Build history of the part. All positions in model axes, mm. Face numbers are marked on the shaded views. A direction names the side the tool comes from. Give positions to 0.01 mm unless a question says otherwise; leave off trailing zeros. Write each loop counter-clockwise with the first axis right and the second up, starting at its lowest first coordinate (ties: lowest second). Pieces come first, ordered by that corner, then holes. Notation, with made-up numbers: M 62.25,-28.5 L 69.25,-28.5 A26 cw 69.25,8.5 Z; hole C -11.75,19 d8. An arc over 180 degrees is marked long. Return JSON: item names as keys, results as strings. Group by question number.
Q1. Band-saw the part on A-A, the plane y = -16.75. Give the cut face in (x, z) (3 decimals), then the cut area to 3 significant figures.
Q2. Band-saw the part on C-C, the plane y = -7.62. Give the cut face in (x, z) (3 decimals), then the cut area to 3 significant figures.
Q3. Band-saw the part on B-B, the plane z = -3.5. Give the cut face in (x, y) (3 decimals).
Q4. Tool access for the marked faces 5 and 6: list every direction of +Z, -Z, +X, -X, +Y, -Y with a clear straight run to the whole face (end or side of a thin tool).
Q5. Band-saw the part on D-D, the plane x = 6. Give the cut face in (y, z).
Q6. Flat gauge pins, fed straight in: pin 1 Ø1.6 at (x, y) = (62, -12.5) entering from -Z; pin 2 Ø1 at (y, z) = (-15, -25.5) entering from -X; pin 3 Ø3 at (y, z) = (-6.5, -34.5) entering from +X (3 decimals). Where does each tip first touch, or does it go through?
Q7. Wall check: probe 1 along X at (y, z) = (-7.62, -9.75); probe 2 along X at (y, z) = (-6.25, -18); probe 3 along Z at (x, y) = (41.5, -1.5). Give the ranges that are in metal, low to high.
Q8. Pull direction Y, two halves, no side cores. Call the marked faces 1, 2, 3 and 4: +Y half, -Y half, draft (parallel to the pull), parting line (faces both ways), or undercut.
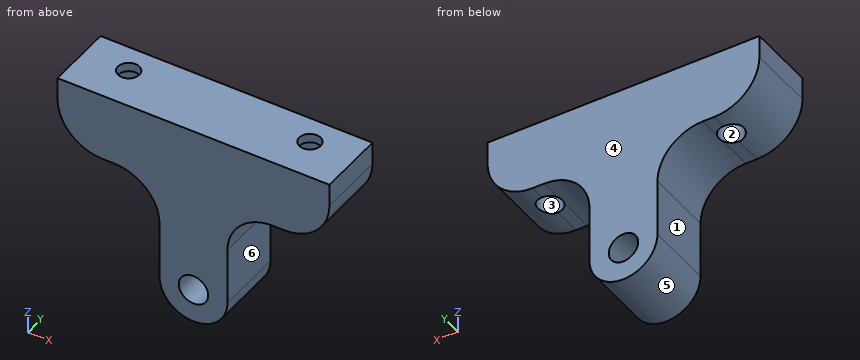
from build123d import *

# Parameters (mm, degrees)
SKETCH1_R               = 4.125
BOSS_EXTRUDE1_DEPTH     = 19.05
SKETCH2_R               = 3
CUT_EXTRUDE1_DEPTH      = 19.05
SKETCH3_R               = 3.44
CUT_EXTRUDE2_DEPTH      = 16.51
CUT_EXTRUDE2_DEPTH_BACK = 16.51


with BuildPart() as part:
    # Sketch1 → Boss-Extrude1 (new body)
    with BuildSketch(Plane(origin=(0, 0, 0), x_dir=(1, 0, 0), z_dir=(0, 1, 0))):
        with BuildLine():
            Line((63.5, 19.05), (60.325, 19.05))
            ThreePointArc((60.325, 19.05), (51.344743879, 22.769743879), (47.625, 31.75))
            Line((47.625, 31.75), (47.625, 47.752))
            ThreePointArc((47.625, 47.752), (38.1, 57.277), (28.575, 47.752))
            Line((28.575, 47.752), (28.575, 31.75))
            ThreePointArc((28.575, 31.75), (24.855256121, 22.769743879), (15.875, 19.05))
            Line((15.875, 19.05), (12.7, 19.05))
            ThreePointArc((12.7, 19.05), (3.719743879, 15.330256121), (0, 6.35))
            Line((0, 6.35), (0, 0))
            Line((0, 0), (76.2, 0))
            Line((76.2, 0), (76.2, 6.35))
            ThreePointArc((76.2, 6.35), (72.480256121, 15.330256121), (63.5, 19.05))
        make_face()
        with Locations(Location((38.1, 47.752, 0), (0, 0, 270))):
            Circle(SKETCH1_R, mode=Mode.SUBTRACT)
    extrude(amount=-BOSS_EXTRUDE1_DEPTH)

    # Sketch2 → Cut-Extrude1 (cut)
    with BuildSketch(Plane(origin=(0, 0, -19.05), x_dir=(-1, 0, 0), z_dir=(0, 0, -1))):
        with Locations((-63.5, -7.62)):
            Circle(SKETCH2_R)
        with Locations((-12.7, -7.62)):
            Circle(SKETCH2_R)
    extrude(amount=-CUT_EXTRUDE1_DEPTH, mode=Mode.SUBTRACT)

    # Sketch3 → Cut-Extrude2 (cut, two sides)
    with BuildSketch(Plane(origin=(0, 0, -19.05), x_dir=(-1, 0, 0), z_dir=(0, 0, -1))) as cut_extrude2_sk:
        with Locations(Location((-63.5, -7.62, 0), (0, 0, 90.000000006))):
            Circle(SKETCH3_R)
        with Locations(Location((-12.7, -7.62, 0), (0, 0, 202.636514893))):
            Circle(SKETCH3_R)
    extrude(amount=CUT_EXTRUDE2_DEPTH, mode=Mode.SUBTRACT)
    extrude(cut_extrude2_sk.sketch, amount=-CUT_EXTRUDE2_DEPTH_BACK, mode=Mode.SUBTRACT)


solid = part.part
From the geometry:
{
 "1": {"outline": "M 0,-6.35 A12.7 ccw 12.7,-19.05 L 15.875,-19.05 A12.7 cw 28.575,-31.75 L 28.575,-47.752 A9.525 ccw 47.625,-47.752 L 47.625,-31.75 A12.7 cw 60.325,-19.05 L 63.5,-19.05 A12.7 ccw 76.2,-6.35 L 76.2,0 L 0,0 Z; hole C 38.1,-47.752 d8.25", "area": "2,090 mm^2"},
 "2": {"outline": "M 0,-6.35 A12.7 ccw 9.26,-18.575 L 9.26,-2.54 L 9.7,-2.54 L 9.7,0 L 0,0 Z; M 15.7,-2.54 L 16.14,-2.54 L 16.14,-19.053 A12.7 cw 28.575,-31.75 L 28.575,-47.752 A9.525 ccw 47.625,-47.752 L 47.625,-31.75 A12.7 cw 60.06,-19.053 L 60.06,-2.54 L 60.5,-2.54 L 60.5,0 L 15.7,0 Z; M 66.5,-2.54 L 66.94,-2.54 L 66.94,-18.575 A12.7 ccw 76.2,-6.35 L 76.2,0 L 66.5,0 Z; hole C 38.1,-47.752 d8.25", "area": "1,830 mm^2"},
 "3": {"outline": "M 0,-19.05 L 76.2,-19.05 L 76.2,0 L 0,0 Z; hole C 12.7,-7.62 d6.88; hole C 63.5,-7.62 d6.88"},
 "4": {"face 5": "-Z, +Y, -Y", "face 6": "-Z, +X, +Y, -Y"},
 "5": {"outline": "M -19.05,-17.14 L 0,-17.14 L 0,0 L -19.05,0 Z"},
 "6": {"pin 1": "stops at z = -19.05", "pin 2": "stops at x = 26.63", "pin 3": "stops at x = 47.625"},
 "7": {"probe 1": "x = 0.46 to 9.26, 16.14 to 60.06, 66.94 to 75.74", "probe 2": "x = 7.64 to 9.54, 15.86 to 60.34, 66.66 to 68.56", "probe 3": "z = -56.65 to -50.09, -45.42 to 0"},
 "8": {"face 1": "draft", "face 2": "undercut", "face 3": "undercut", "face 4": "+Y half"}
}
